```python
from build123d import *

# Parameters (mm, degrees)
SKETCH1_W                      = 56.83
SKETCH1_H                      = 16
SKETCH1_R                      = 2
BASE_FLANGE1_DEPTH             = 1.5875
EDGE_FLANGE1_STRIP_W           = 7.8232
EDGE_FLANGE1_STRIP_H           = 1.5875
EDGE_FLANGE1_STRIP_CUT_DEPTH   = 16
EDGE_FLANGE1_STRIP_2_W         = 7.8232
EDGE_FLANGE1_STRIP_2_H         = 1.5875
EDGE_FLANGE1_STRIP_CUT_2_DEPTH = 16
EDGE_FLANGE1_DEPTH             = 16
EDGE_FLANGE1_BEND_DEPTH        = 16
SKETCH12_R                     = 2
CUT_EXTRUDE1_DEPTH             = 61.773094839


# Sheet-metal steps are written as plain solids
with BuildPart() as part:
    # Sketch1 → Base-Flange1 (new body)
    with BuildSketch(Plane(origin=(0, 0, 0), x_dir=(1, 0, 0), z_dir=(0, 1, 0))):
        with Locations((28.415, 8)):
            Rectangle(SKETCH1_W, SKETCH1_H)
        with Locations(Location((28.415, 8, 0), (0, 0, 270))):
            Circle(SKETCH1_R, mode=Mode.SUBTRACT)
    extrude(amount=-BASE_FLANGE1_DEPTH)

    # Edge-Flange1 strip (across the edge) → Edge-Flange1 strip cut (cut)
    with BuildSketch(Plane(origin=(56.83, 0, 0), x_dir=(-1, 0, 0), z_dir=(0, 0, -1))):
        with Locations((-1.5875, -0.79375)):
            Rectangle(EDGE_FLANGE1_STRIP_W, EDGE_FLANGE1_STRIP_H)
    extrude(amount=EDGE_FLANGE1_STRIP_CUT_DEPTH, mode=Mode.SUBTRACT)

    # Edge-Flange1 strip 2 (across the edge) → Edge-Flange1 strip cut 2 (cut)
    with BuildSketch(Plane.XY.offset(-16)):
        with Locations((-1.5875, -0.79375)):
            Rectangle(EDGE_FLANGE1_STRIP_2_W, EDGE_FLANGE1_STRIP_2_H)
    extrude(amount=EDGE_FLANGE1_STRIP_CUT_2_DEPTH, mode=Mode.SUBTRACT)

    # Edge-Flange1 section (across the edge) → Edge-Flange1 (add)
    with BuildSketch(Plane(origin=(56.83, 0, 0), x_dir=(-1, 0, 0), z_dir=(0, 0, -1))):
        with BuildLine():
            Line((0, 0.7366), (0, 14.4125))
            Line((0, 14.4125), (1.5875, 14.4125))
            Line((1.5875, 14.4125), (1.5875, 0.7366))
            ThreePointArc((1.5875, 0.7366), (1.803245145, 0.215745145), (2.3241, 0))
            Line((2.3241, 0), (2.3241, -1.5875))
            ThreePointArc((2.3241, -1.5875), (0.68071313, -0.90678687), (0, 0.7366))
        make_face()
    extrude(amount=EDGE_FLANGE1_DEPTH)

    # Edge-Flange1 section 2 (across the edge) → Edge-Flange1 bend (add)
    with BuildSketch(Plane.XY.offset(-16)):
        with BuildLine():
            Line((0, 0.7366), (0, 14.4125))
            Line((0, 14.4125), (1.5875, 14.4125))
            Line((1.5875, 14.4125), (1.5875, 0.7366))
            ThreePointArc((1.5875, 0.7366), (1.803245145, 0.215745145), (2.3241, 0))
            Line((2.3241, 0), (2.3241, -1.5875))
            ThreePointArc((2.3241, -1.5875), (0.68071313, -0.90678687), (0, 0.7366))
        make_face()
    extrude(amount=EDGE_FLANGE1_BEND_DEPTH)

    # Sketch12 → Cut-Extrude1 (cut, through all)
    with BuildSketch(Plane(origin=(56.83, 0, 0), x_dir=(0, 0, -1), z_dir=(1, 0, 0))):
        with Locations(Location((8, 7.57455, 0), (0, 0, 90))):
            Circle(SKETCH12_R)
    extrude(amount=-CUT_EXTRUDE1_DEPTH, mode=Mode.SUBTRACT)


solid = part.part
```
Source: CAD feature listing. Evaluate the final solid. Frame: model axes, mm. A direction names the side the tool comes from. Round coordinates to 2 decimals unless told otherwise and drop trailing zeros. Write each loop counter-clockwise with the first axis right and the second up, starting at its lowest first coordinate (ties: lowest second). Pieces come first, ordered by that corner, then holes. Notation, with made-up numbers: M -36,35.5 L 17,35.5 A18 ccw 17,57.5 Z; hole C 55,71 d3. An arc over 180 degrees is marked long. Answer as a JSON object with one key per item and string values. Group by question number.
(1) Section query C-C on x = 29. Output: boundary loops of the cut face in (y, z), then the cut area to 3 significant figures.
(2) Reachability of faces 5 (the flat face through (1.588, 6, -10)), 6 (the flat face through (1, 14.412, -8)) from +Z, -Z, +X, -X, +Y, -Y: full face, straight path, thin tool, end or side. Return the list, or none.
(3) Ray query, line 1 (X direction, y = 4, z = -2); line 2 (Y direction, x = 37.5, z = -4.75); line 3 (X direction, y = -0.8, z = -8) (3 decimals). Return the intervals inside material, ascending. Write a range as [from, to].
(4) First-contact query: pin 1 (5 mm diameter, centred on x = 28.415, z = -8, fed in from -Y); pin 2 (4 mm diameter, centred on x = 48, z = -14, fed in from +Y). Flat tips, straight axial feed; report the tip coordinate or a pass-through.
(5) Section query A-A on z = -8. Output: boundary loops of the cut face in (x, y) (1 decimal).
(6) Section query B-B on y = 11.75. Output: boundary loops of the cut face in (x, z), then the cut area to 3 significant figures.
(7) Mould query, pull axis X, two halves, no side actions, for faces 1 (the flat face through (55.242, 6, -6)), 2 (the flat face through (28, 0, -5)), 3 (the cylindrical face through (56.131, -0.925, -7.888)), 4 (the cylindrical face through (0.8, 6.1, -6.65)). Classes: +X half, -X half, draft (parallel to the pull), parting line (faces both ways), or undercut.
(8) Section query D-D on y = 8.5. Output: boundary loops of the cut face in (x, z).
Computed values:
{
 "1": {"outline": "M -1.59,-16 L 0,-16 L 0,-9.91 L -1.59,-9.91 Z; M -1.59,-6.09 L 0,-6.09 L 0,0 L -1.59,0 Z", "area": "19.3 mm^2"},
 "2": {"face 5": "+Z, -Z, +Y", "face 6": "+Z, -Z, +X, -X, +Y"},
 "3": {"line 1": "[0, 1.59], [55.24, 56.83]", "line 2": "[-1.59, 0]", "line 3": "[0.58, 26.415], [30.415, 56.25]"},
 "4": {"pin 1": "y = -1.59", "pin 2": "y = 0"},
 "5": {"outline": "M 0,0.7 A2.3 ccw 2.3,-1.6 L 26.4,-1.6 L 26.4,0 L 2.3,0 A0.7 cw 1.6,0.7 L 1.6,5.6 L 0,5.6 Z; M 0,9.6 L 1.6,9.6 L 1.6,14.4 L 0,14.4 Z; M 30.4,-1.6 L 54.5,-1.6 A2.3 ccw 56.8,0.7 L 56.8,5.6 L 55.2,5.6 L 55.2,0.7 A0.7 cw 54.5,0 L 30.4,0 Z; M 55.2,9.6 L 56.8,9.6 L 56.8,14.4 L 55.2,14.4 Z"},
 "6": {"outline": "M 0,-16 L 1.59,-16 L 1.59,0 L 0,0 Z; M 55.24,-16 L 56.83,-16 L 56.83,0 L 55.24,0 Z", "area": "50.8 mm^2"},
 "7": {"face 1": "undercut", "face 2": "undercut", "face 3": "+X half", "face 4": "draft"},
 "8": {"outline": "M 0,-16 L 1.59,-16 L 1.59,-9.77 L 0,-9.77 Z; M 0,-6.23 L 1.59,-6.23 L 1.59,0 L 0,0 Z; M 55.24,-16 L 56.83,-16 L 56.83,-9.77 L 55.24,-9.77 Z; M 55.24,-6.23 L 56.83,-6.23 L 56.83,0 L 55.24,0 Z"}
}
